```python
from build123d import *

# Parameters (mm, degrees)
SKETCH1_W           = 26
SKETCH1_H           = 26
SKETCH1_R           = 1.55
BOSS_EXTRUDE1_DEPTH = 1.6
SKETCH2_W           = 4.4
SKETCH2_H           = 6
BOSS_EXTRUDE2_DEPTH = 3.5
SKETCH3_W           = 3
SKETCH3_H           = 2.6
BOSS_EXTRUDE3_DEPTH = 1


with BuildPart() as part:
    # Sketch1 → Boss-Extrude1 (new body)
    with BuildSketch(Plane(origin=(0, 0, 0), x_dir=(1, 0, 0), z_dir=(0, 1, 0))):
        Rectangle(SKETCH1_W, SKETCH1_H)
        with Locations((-10, 10)):
            Circle(SKETCH1_R, mode=Mode.SUBTRACT)
        with Locations((10, 10)):
            Circle(SKETCH1_R, mode=Mode.SUBTRACT)
        with Locations((10, -10)):
            Circle(SKETCH1_R, mode=Mode.SUBTRACT)
        with Locations((-10, -10)):
            Circle(SKETCH1_R, mode=Mode.SUBTRACT)
    extrude(amount=BOSS_EXTRUDE1_DEPTH)

    # Sketch2 → Boss-Extrude2 (add)
    with BuildSketch(Plane(origin=(0, 1.6, 0), x_dir=(1, 0, 0), z_dir=(0, 1, 0))):
        with Locations((-10.2, 0)):
            Rectangle(SKETCH2_W, SKETCH2_H)
        with Locations((10.2, 0)):
            Rectangle(SKETCH2_W, SKETCH2_H)
    extrude(amount=BOSS_EXTRUDE2_DEPTH)

    # Sketch3 → Boss-Extrude3 (add)
    with BuildSketch(Plane(origin=(0, 1.6, 0), x_dir=(1, 0, 0), z_dir=(0, 1, 0))):
        Rectangle(SKETCH3_W, SKETCH3_H)
    extrude(amount=BOSS_EXTRUDE3_DEPTH)


solid = part.part
```
The listing builds one solid part. Answer for the finished solid, in the listing's coordinates (mm). A direction names the side the tool comes from. Give positions to 0.01 mm unless a question says otherwise; leave off trailing zeros. Loops run counter-clockwise (first coordinate to the right, second up) from the corner with the lowest first, then second, coordinate; pieces in that order, holes last. Notation, with made-up numbers: M -12,-2 L 14,-2 A4 ccw 14,4 Z; hole C 45.25,-10 d9. An arc over 180 degrees is marked long. One line per item, written item: value.
1. For faces 1 (the face through (0, 2, -1.3)), 2 (the face through (1.5, 2, 0)), 3 (the face through (10, 3, 3)), determine the directions among +Z, -Z, +X, -X, +Y, -Y from which every point of the face is accessible in a straight line to the end or side of a thin tool.
Found:
face 1: -Z, +Y
face 2: +Z, -Z, +Y
face 3: +Z, +X, -X, +Y
2. Section B-B on x = 10 is taken. Determine the outline of the cut face in (y, z).
Found:
outline: M 0,-13 L 1.6,-13 L 1.6,-11.55 L 0,-11.55 Z; M 0,-8.45 L 1.6,-8.45 L 1.6,-3 L 5.1,-3 L 5.1,3 L 1.6,3 L 1.6,8.45 L 0,8.45 Z; M 0,11.55 L 1.6,11.55 L 1.6,13 L 0,13 Z
3. Section A-A on z = -10 is taken. Determine the outline of the cut face in (x, y).
Found:
outline: M -13,0 L -11.55,0 L -11.55,1.6 L -13,1.6 Z; M -8.45,0 L 8.45,0 L 8.45,1.6 L -8.45,1.6 Z; M 11.55,0 L 13,0 L 13,1.6 L 11.55,1.6 Z
4. Section C-C on y = 0.3 is taken. Determine the outline of the cut face in (x, z), plus the area to 3 significant figures.
Found:
outline: M -13,-13 L 13,-13 L 13,13 L -13,13 Z; hole C -10,-10 d3.1; hole C -10,10 d3.1; hole C 10,-10 d3.1; hole C 10,10 d3.1
area: 646 mm^2
5. For a pull along X with two mould halves and no side action, classify faces 4 (the face through (0, 2, 1.3)), 5 (the face through (12.4, 3, 0)), 6 (the face through (0, 1, -13)) as pulls with the +X half, pulls with the -X half, needs draft (parallel to the pull), parting line crosses it, or undercut.
Found:
face 4: undercut
face 5: pulls with the +X half
face 6: needs draft
6. Find the intervals of material crossed by probe 1 along Z at (x, y) = (10, 0.5); probe 2 along X at (y, z) = (4.1, 2.5), in increasing order.
Found:
probe 1: -13 to -11.55, -8.45 to 8.45, 11.55 to 13
probe 2: -12.4 to -8, 8 to 12.4
7. Each of these flat-tipped pins is pushed along its axis until it touches: P1, Ø1, axis at x = -9.5, y = 3, coming from the -Z side; P2, Ø1, axis at y = 4, z = 0, coming from the -X side; P3, Ø0.5, axis at x = 0, y = 2, coming from the -Z side. Where does it stop, or does it pass through?
Found:
P1: z = -3
P2: x = -12.4
P3: z = -1.3
8. Section D-D on x = 2.5 is taken. Determine the outline of the cut face in (y, z).
Found:
outline: M 0,-13 L 1.6,-13 L 1.6,13 L 0,13 Z
